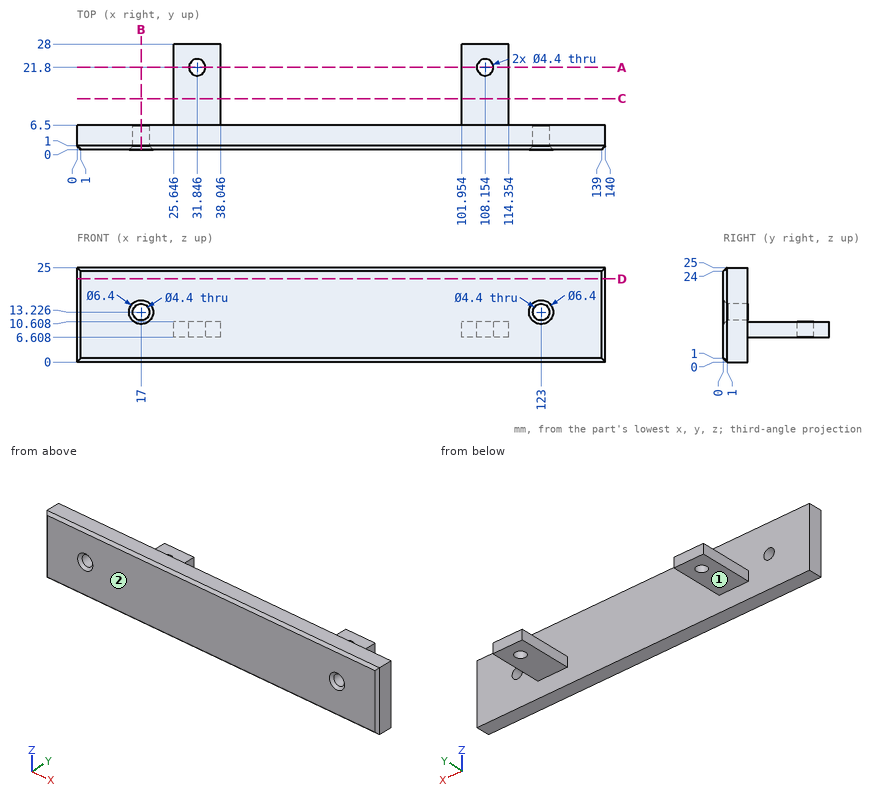
Could you check a few things on this drawing? It's one solid part, dimensions in mm from its lowest x, y, z. A direction names the side the tool comes from. Coordinates: 2 decimals unless noted, no trailing zeros. Order: outer loops, then holes, each group sorted by start corner. A loop starts at its lowest first (then second) coordinate and runs counter-clockwise, first axis right, second up. Notation, with made-up numbers: (-11, -15.75) -> (28, -15.75) arc R34 cw to (28, 18.25) -> close; hole circle Ø9 at (41.25, -0.5). An arc over 180 degrees is marked (long way). Answer in a Markdown table with one row per item.
(1) Please list where these lines run through material, in increasing order: probe 1 along Z at (x, y) = (17, 3.9); probe 2 along Y at (x, z) = (108, 7); probe 3 along X at (y, z) = (17, 10).
Answer key:
| item | result |
|---|---|
| probe 1 | 0 to 11.03, 15.43 to 25 |
| probe 2 | 0 to 19.61, 23.99 to 28 |
| probe 3 | 25.65 to 38.05, 101.95 to 114.35 |
(2) Will these pins go through, and if not, where does the flat tip stop? pin 1 Ø4 at (y, z) = (21.5, 12) entering from -X; pin 2 Ø6 at (x, y) = (47.5, 8) entering from -Z; pin 3 Ø13.5 at (x, y) = (32, 17) entering from +Z; pin 4 Ø2.5 at (x, y) = (108.154, 21.8) entering from -Z.
Answer key:
| item | result |
|---|---|
| pin 1 | x = 25.65 |
| pin 2 | z = 0 |
| pin 3 | z = 10.61 |
| pin 4 | through |
(3) I want a section at B-B on x = 17. List the corners of the cut face in (y, z) for me.
Answer key:
| item | result |
|---|---|
| outline | (0, 1) -> (1, 0) -> (6.5, 0) -> (6.5, 11.03) -> (1, 11.03) -> (0, 10.03) -> close; (0, 16.43) -> (1, 15.43) -> (6.5, 15.43) -> (6.5, 25) -> (1, 25) -> (0, 24) -> close |
(4) I want a section at D-D on z = 22. List the corners of the cut face in (x, y) for me, then the cut area to 3 significant figures.
Answer key:
| item | result |
|---|---|
| outline | (0, 1) -> (1, 0) -> (139, 0) -> (140, 1) -> (140, 6.5) -> (0, 6.5) -> close |
| area | 909 mm^2 |
(5) I want a section at C-C on y = 13.5. List the corners of the cut face in (x, z) for me.
Answer key:
| item | result |
|---|---|
| outline | (25.65, 6.61) -> (38.05, 6.61) -> (38.05, 10.61) -> (25.65, 10.61) -> close; (101.95, 6.61) -> (114.35, 6.61) -> (114.35, 10.61) -> (101.95, 10.61) -> close |
(6) I want a section at A-A on y = 21.8. List the corners of the cut face in (x, z) for me.
Answer key:
| item | result |
|---|---|
| outline | (25.65, 6.61) -> (29.65, 6.61) -> (29.65, 10.61) -> (25.65, 10.61) -> close; (34.05, 6.61) -> (38.05, 6.61) -> (38.05, 10.61) -> (34.05, 10.61) -> close; (101.95, 6.61) -> (105.95, 6.61) -> (105.95, 10.61) -> (101.95, 10.61) -> close; (110.35, 6.61) -> (114.35, 6.61) -> (114.35, 10.61) -> (110.35, 10.61) -> close |
(7) On a 3-axis mill with a long thin cutter (end or side, diameter ignored), from which of +Z, -Z, +X, -X, +Y, -Y can I reach the whole of each face in a straight line? I mean the marked faces 1 and 2. Say none if no direction works.
Answer key:
| item | result |
|---|---|
| face 1 | -Z, +X, -X, +Y |
| face 2 | +Z, -Z, +X, -X, -Y |
